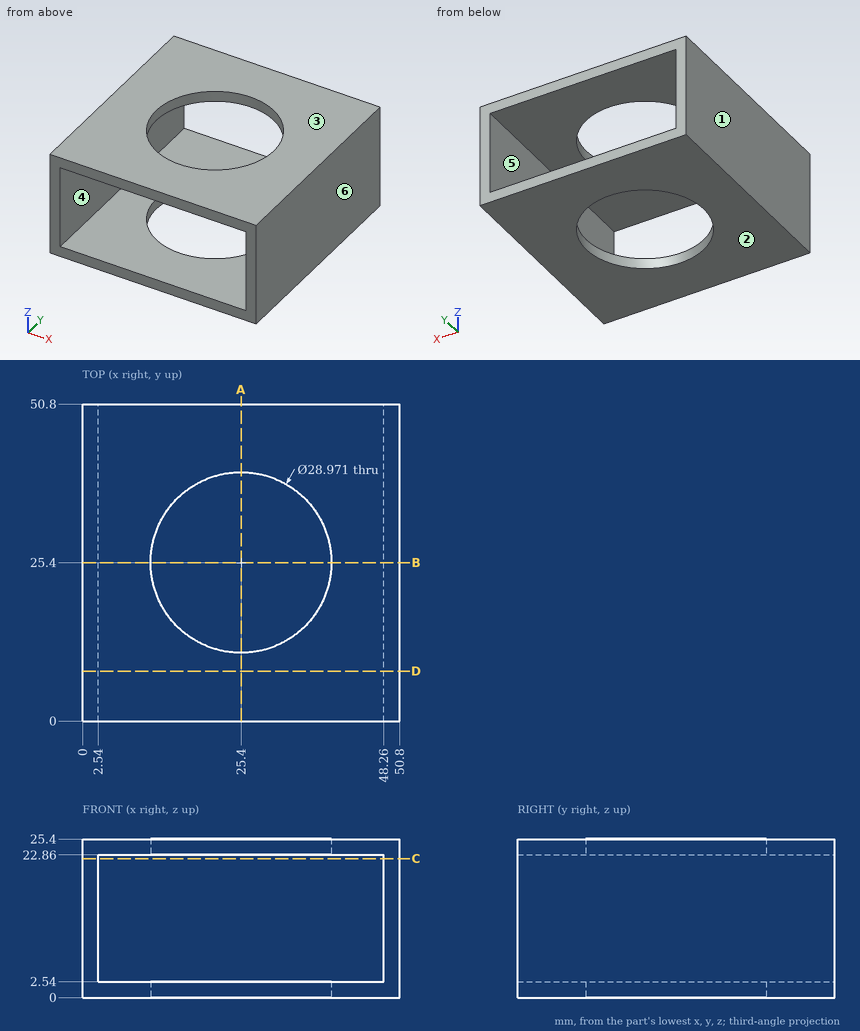
Source: three-view drawing plus pictorial views. Frame: mm from the lowest corner of the part. A direction names the side the tool comes from. Round coordinates to 2 decimals unless told otherwise and drop trailing zeros. Write each loop counter-clockwise with the first axis right and the second up, starting at its lowest first coordinate (ties: lowest second). Pieces come first, ordered by that corner, then holes. Notation, with made-up numbers: M 66,42 L 98,42 A15 cw 98,58 Z; hole C 19.5,60 d10. An arc over 180 degrees is marked long. Write item = value, one per line.
Item 1: Material intervals for line 1 along Z through (x, y) = (36.5, 48); line 2 along X through (y, z) = (39.5, 21); line 3 along Y through (x, z) = (25.4, 1.1), sorted ascending. Write a range as [from, to].
Findings:
line_1 = [0, 2.54], [22.86, 25.4]
line_2 = [0, 2.54], [48.26, 50.8]
line_3 = [0, 10.91], [39.89, 50.8]
Item 2: Section query C-C on z = 22.25. Return loops of the section in (x, y), then the cut area to 3 significant figures.
Findings:
outline = M 0,0 L 2.54,0 L 2.54,50.8 L 0,50.8 Z; M 48.26,0 L 50.8,0 L 50.8,50.8 L 48.26,50.8 Z
area = 258 mm^2
Item 3: Access query for the marked faces 5 and 6. Directions: +Z, -Z, +X, -X, +Y, -Y. A direction counts if a zero-diameter tool reaches every point of the face in a straight line with its end or side. Return the directions, or none.
Findings:
face_5 = +Y, -Y
face_6 = +Z, -Z, +X, +Y, -Y
Item 4: Section query D-D on y = 8. Return loops of the section in (x, z).
Findings:
outline = M 0,0 L 50.8,0 L 50.8,25.4 L 0,25.4 Z; hole M 2.54,2.54 L 48.26,2.54 L 48.26,22.86 L 2.54,22.86 Z
Item 5: Pin query (flat end, axial travel): P1, Ø6, axis at y = 37, z = 16.5, coming from the -X side. Return the tip coordinate at first contact, or that it passes through.
Findings:
P1 = 0
Item 6: Section query A-A on x = 25.4. Return loops of the section in (y, z).
Findings:
outline = M 0,0 L 10.91,0 L 10.91,2.54 L 0,2.54 Z; M 0,22.86 L 10.91,22.86 L 10.91,25.4 L 0,25.4 Z; M 39.89,0 L 50.8,0 L 50.8,2.54 L 39.89,2.54 Z; M 39.89,22.86 L 50.8,22.86 L 50.8,25.4 L 39.89,25.4 Z
Item 7: Pull-direction query (Z, two-part tool) for the marked faces 1, 2, 3 and 4; classes: pulls with the +Z half, pulls with the -Z half, needs draft (parallel to the pull), parting line crosses it, or undercut.
Findings:
face_1 = needs draft
face_2 = pulls with the -Z half
face_3 = pulls with the +Z half
face_4 = undercut
Item 8: Section query B-B on y = 25.4. Return loops of the section in (x, z), then the cut area to 3 significant figures.
Findings:
outline = M 0,0 L 10.91,0 L 10.91,2.54 L 2.54,2.54 L 2.54,22.86 L 10.91,22.86 L 10.91,25.4 L 0,25.4 Z; M 39.89,0 L 50.8,0 L 50.8,25.4 L 39.89,25.4 L 39.89,22.86 L 48.26,22.86 L 48.26,2.54 L 39.89,2.54 Z
area = 214 mm^2
